Part model, mm, in its own coordinate system. A direction names the side the tool comes from. Coordinates: 2 decimals unless noted, no trailing zeros. Loops run counter-clockwise (first coordinate to the right, second up) from the corner with the lowest first, then second, coordinate; pieces in that order, holes last. Notation, with made-up numbers: (50.25, 77.5) - (94.25, 77.5) arc R6 ccw to (94.25, 85.5) - close; hole circle Ø11 at (88.25, 68). An arc over 180 degrees is marked (long way). Use a Markdown table: item, result. Add a question column.
1) Band-saw the part on B-B (z = 7.75). Give the cut face in (x, y).
2) Drop flat-ended pins along their axis: P1, Ø6.5, axis at x = 0, y = -12, coming from the -Z side; P2, Ø2, axis at x = -0.5, y = -12, coming from the -Z side; P3, Ø3, axis at x = 4, z = 9.5, coming from the +Y side; P4, Ø4.5, axis at y = -7, z = 9.5, coming from the +X side. Give the stop position or say it passes through.
3) Tool access for faces 1 (the face through (0, 12.952, 9)), 2 (the face through (-4.563, -17.102, 8.972)), 3 (the face through (-11, 1, 7)): list every direction of +Z, -Z, +X, -X, +Y, -Y with a clear straight run to the whole face (end or side of a thin tool).
4) Band-saw the part on A-A (y = 8). Give the cut face in (x, z).
5) Pull direction X, two halves, no side cores. Call faces 4 (the face through (17.3, -2, 3)), 5 (the face through (-8.529, -19.326, 3.451)), 6 (the face through (-0.81, 9.55, 7.06)), 7 (the face through (0.228, -13.735, 7.056)): +X half, -X half, draft (parallel to the pull), parting line (faces both ways), or undercut.
6) Probe probe 1 along Y at (x, z) = (0, 7.75); probe 2 along Y at (x, z) = (-3, 1); probe 3 along X at (y, z) = (-12, 4.5). List the from-to ranges inside material, lowest first. Write a range as [from, to].
7) Band-saw the part on D-D (z = 1). Give the cut face in (x, y).
from build123d import *

# Parameters (mm, degrees)
ESBO_O1_W                = 34.6
ESBO_O1_H                = 26
RESSALTO_EXTRUS_O1_DEPTH = 7
ESBO_O10_W               = 34.6
ESBO_O10_H               = 2.5
RESSALTO_EXTRUS_O4_DEPTH = 7
CHANFRO1_SIZE            = 7
CHANFRO2_SIZE2           = 7
CHANFRO2_SIZE            = 2.54779164
RESSALTO_EXTRUS_O5_DEPTH = 4
ESBO_O11_R               = 1.75
CORTE_EXTRUS_O1_DEPTH    = 34.504328079
ESBO_O12_R               = 3.5
CORTE_EXTRUS_O2_DEPTH    = 3


with BuildPart() as part:
    # Esboço1 → Ressalto-extrusão1 (new body)
    with BuildSketch(Plane.XY):
        Rectangle(ESBO_O1_W, ESBO_O1_H)
    extrude(amount=RESSALTO_EXTRUS_O1_DEPTH)

    # Esboço10 → Ressalto-extrusão4 (add)
    with BuildSketch(Plane(origin=(0, 0, 0), x_dir=(-1, 0, 0), z_dir=(0, 0, -1))):
        Polygon((-17.3, -19.5), (0, -26.5), (17.3, -19.5), (17.3, -13), (-17.3, -13), align=None)
        with Locations((0, 14.25)):
            Rectangle(ESBO_O10_W, ESBO_O10_H)
    extrude(amount=-RESSALTO_EXTRUS_O4_DEPTH)

    # Chanfro1
    chanfro1_edges = [part.edges().sort_by_distance(p)[0] for p in [
        (8.65, -23, 7),
        (-8.65, -23, 7),
    ]]
    chamfer(chanfro1_edges, length=CHANFRO1_SIZE - 0.0001)  # a hair under: the kernel refuses the full size

    # Chanfro2
    chanfro2_edges = [part.edges().sort_by_distance(p)[0] for p in [
        (0, 15.5, 7),
    ]]
    chanfro2_side = [part.faces().sort_by_distance(p)[0] for p in [
        (0, 15.449044167, 7),
    ]]
    chamfer(chanfro2_edges, length=CHANFRO2_SIZE - 0.0001, length2=CHANFRO2_SIZE2 - 0.0001, reference=chanfro2_side[0])  # a hair under: the kernel refuses the full size

    # Esboço13 → Ressalto-extrusão5 (add)
    with BuildSketch(Plane.XY.offset(7)):
        Polygon((9, -15.307069068), (9, 12.95220836), (-9, 12.95220836), (-9, -15.307069068), (0, -18.948687565), align=None)
    extrude(amount=RESSALTO_EXTRUS_O5_DEPTH)

    # Esboço11 → Corte-extrusão1 (cut, through all)
    with BuildSketch(Plane.XY.offset(11)):
        with Locations(Location((0, -12, 0), (0, 0, 180))):
            Circle(ESBO_O11_R)
        with Locations(Location((0, 8, 0), (0, 0, 180))):
            Circle(ESBO_O11_R)
    extrude(amount=-CORTE_EXTRUS_O1_DEPTH, mode=Mode.SUBTRACT)

    # Esboço12 → Corte-extrusão2 (cut)
    with BuildSketch(Plane(origin=(0, 0, 0), x_dir=(-1, 0, 0), z_dir=(0, 0, -1))):
        with Locations((0, 8)):
            Circle(ESBO_O12_R)
        with Locations((0, -12)):
            Circle(ESBO_O12_R)
    extrude(amount=-CORTE_EXTRUS_O2_DEPTH, mode=Mode.SUBTRACT)


solid = part.part
Answer block:
| question | item | result |
|---|---|---|
| 1 | outline | (-9, -15.31) - (0, -18.95) - (9, -15.31) - (9, 12.95) - (-9, 12.95) - close; hole circle Ø3.5 at (0, -12); hole circle Ø3.5 at (0, 8) |
| 2 | P1 | z = 3 |
| 2 | P2 | through |
| 2 | P3 | y = 12.95 |
| 2 | P4 | x = 9 |
| 3 | face 1 | +Z, +X, -X, +Y |
| 3 | face 2 | +Z, -X, -Y |
| 3 | face 3 | +Z, +Y, -Y |
| 4 | outline | (-17.3, 0) - (-3.5, 0) - (-3.5, 3) - (-1.75, 3) - (-1.75, 11) - (-9, 11) - (-9, 7) - (-17.3, 7) - close; (1.75, 3) - (3.5, 3) - (3.5, 0) - (17.3, 0) - (17.3, 7) - (9, 7) - (9, 11) - (1.75, 11) - close |
| 5 | face 4 | +X half |
| 5 | face 5 | -X half |
| 5 | face 6 | undercut |
| 5 | face 7 | undercut |
| 6 | probe 1 | [-18.95, -13.75], [-10.25, 6.25], [9.75, 12.95] |
| 6 | probe 2 | [-24.21, -13.8], [-10.2, 6.2], [9.8, 15.14] |
| 6 | probe 3 | [-17.3, -1.75], [1.75, 17.3] |
| 7 | outline | (-17.3, -18.42) - (0, -25.42) - (17.3, -18.42) - (17.3, 15.14) - (-17.3, 15.14) - close; hole circle Ø7 at (0, -12); hole circle Ø7 at (0, 8) |
